Part print with two shaded views. Sizes in mm from the minimum x, y, z corner. A direction names the side the tool comes from. Round coordinates to 2 decimals unless told otherwise and drop trailing zeros. Write each loop counter-clockwise with the first axis right and the second up, starting at its lowest first coordinate (ties: lowest second). Pieces come first, ordered by that corner, then holes.
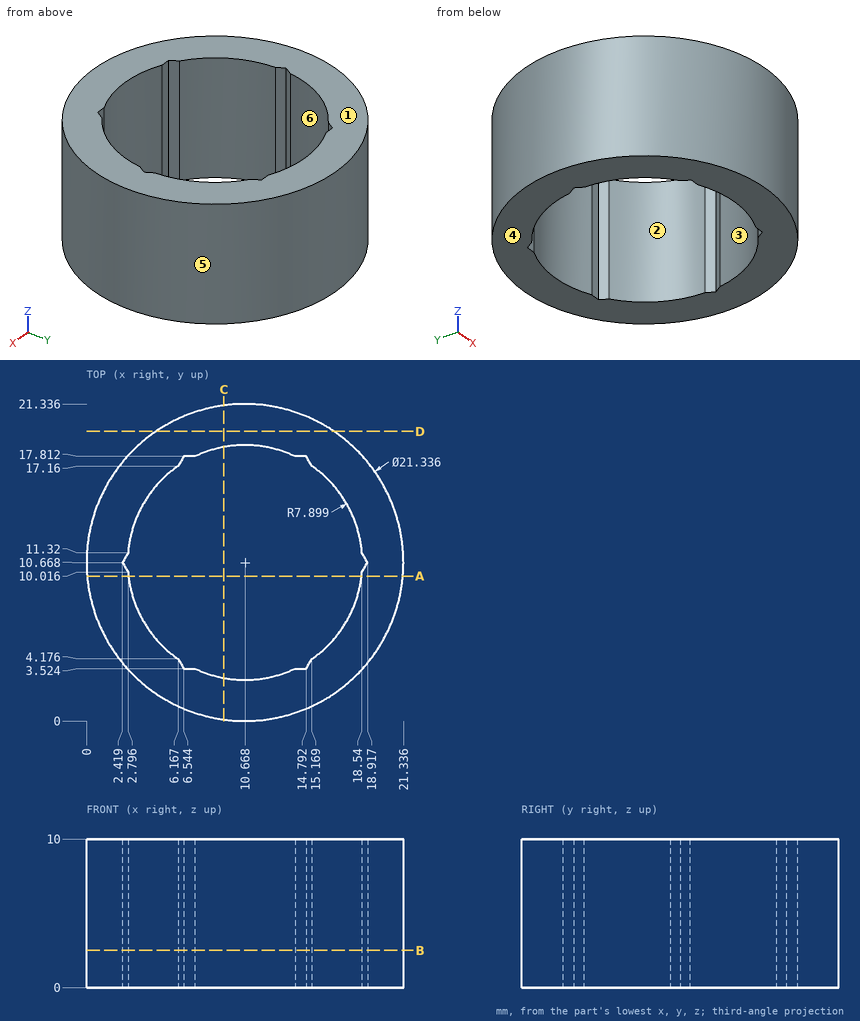
Q1. Which spindle directions (+Z, -Z, +X, -X, +Y, -Y) get a long thin tool onto all of the face, cutting with end or side? Do the marked faces 1 and 2. Say none if no direction does.
Values follow:
face 1: +Z, +X, -X, +Y, -Y
face 2: +Z, -Z
Q2. Cut at B-B on z = 2.5. Write the cut outline in (x, y) (1 decimal), plus the area to 3 significant figures.
Values follow:
outline: circle Ø21.3 at (10.7, 10.7); hole (2.4, 10.7) - (2.8, 10) arc R7.9 ccw to (6.2, 4.2) - (6.5, 3.5) - (7.3, 3.5) arc R7.9 ccw to (14, 3.5) - (14.8, 3.5) - (15.2, 4.2) arc R7.9 ccw to (18.5, 10) - (18.9, 10.7) - (18.5, 11.3) arc R7.9 ccw to (15.2, 17.2) - (14.8, 17.8) - (14, 17.8) arc R7.9 ccw to (7.3, 17.8) - (6.5, 17.8) - (6.2, 17.2) arc R7.9 ccw to (2.8, 11.3) - close
area: 160 mm2
Q3. Cut at D-D on y = 19.5. Write the cut outline in (x, z) (1 decimal).
Values follow:
outline: (4.7, 0) - (16.7, 0) - (16.7, 10) - (4.7, 10) - close
Q4. Cut at C-C on x = 9.25. Write the cut outline in (y, z) (1 decimal).
Values follow:
outline: (0.1, 0) - (2.9, 0) - (2.9, 10) - (0.1, 10) - close; (18.4, 0) - (21.2, 0) - (21.2, 10) - (18.4, 10) - close
Q5. Wall check: L1, parallel to X at y = 8.5, z = 5.5 (1 decimal); L2, parallel to X at y = 7.5, z = 2 (1 decimal); L3, parallel to Y at x = 15.25, z = 4.75 (1 decimal). Give the ranges that are in metal, low to high.
Values follow:
L1: x = 0.2 to 3.1, 18.3 to 21.1
L2: x = 0.5 to 3.4, 17.9 to 20.9
L3: y = 1 to 4.2, 17.1 to 20.3
Q6. Drop flat-ended pins along their axis: pin 1 (0.6 mm diameter, centred on x = 7, z = 5, fed in from +Y); pin 2 (4 mm diameter, centred on y = 15.5, z = 2.5, fed in from +X); pin 3 (2 mm diameter, centred on y = 15, z = 2, fed in from -X). Give the stop position or say it passes through.
Values follow:
pin 1: stops at y = 20.79
pin 2: stops at x = 20.95
pin 3: stops at x = 0.53
Q7. Mould opens along X. For the marked faces 3, 4, 5 and 6 say: +X half, -X half, draft (parallel to the pull), parting line (faces both ways), or undercut.
Values follow:
face 3: undercut
face 4: draft
face 5: parting line
face 6: undercut
Q8. Cut at A-A on y = 9.75. Write the cut outline in (x, z).
Values follow:
outline: (0.04, 0) - (2.82, 0) - (2.82, 10) - (0.04, 10) - close; (18.51, 0) - (21.3, 0) - (21.3, 10) - (18.51, 10) - close
